```python
from build123d import *

# Parameters (mm, degrees)
HOLE_WIZARD_M32_D           = 2.5
HOLE_WIZARD_M32_DEPTH       = 8.5
HOLE_WIZARD_M32_CSINK_D     = 3.05
HOLE_WIZARD_M32_CSINK_ANGLE = 120
HOLE_WIZARD_M32_TIP         = 0.751075774
HOLE_WIZARD_1_D             = 3.3
HOLE_WIZARD_1_DEPTH         = 6
HOLE_WIZARD_1_CSINK_D       = 4.05
HOLE_WIZARD_1_CSINK_ANGLE   = 120
HOLE_WIZARD_1_TIP           = 0.991420021


with BuildPart() as part:
    # Эскиз2 → Повернуть1 (revolve)
    with BuildSketch(Plane(origin=(0, 0, 0), x_dir=(0, 0, -1), z_dir=(1, 0, 0))):
        Polygon((0, 0), (2, 0), (2, 0.01), (3, 0.01), (3, 8.01), (2, 8.01), (2, 25.01), (0, 25.01), align=None)
    revolve(axis=Axis((0, 0, 0), (0, 1, 0)))

    # Отверстие обработанное метчиком M32
    with Locations(Plane(origin=(0, 25.01, 0), x_dir=(-1, 0, 0), z_dir=(0, 1, 0))):
        with Locations((0, 0)):
            CounterSinkHole(HOLE_WIZARD_M32_D / 2, HOLE_WIZARD_M32_CSINK_D / 2, depth=HOLE_WIZARD_M32_DEPTH, counter_sink_angle=HOLE_WIZARD_M32_CSINK_ANGLE)
            with Locations((0, 0, -(HOLE_WIZARD_M32_DEPTH + HOLE_WIZARD_M32_TIP / 2))):  # 118° drill point
                Cone(0, HOLE_WIZARD_M32_D / 2, HOLE_WIZARD_M32_TIP, mode=Mode.SUBTRACT)

    # Отверстие обработанное метчиком 1
    with Locations(Plane.XZ):
        with Locations((0, 0)):
            CounterSinkHole(HOLE_WIZARD_1_D / 2, HOLE_WIZARD_1_CSINK_D / 2, depth=HOLE_WIZARD_1_DEPTH, counter_sink_angle=HOLE_WIZARD_1_CSINK_ANGLE)
            with Locations((0, 0, -(HOLE_WIZARD_1_DEPTH + HOLE_WIZARD_1_TIP / 2))):  # 118° drill point
                Cone(0, HOLE_WIZARD_1_D / 2, HOLE_WIZARD_1_TIP, mode=Mode.SUBTRACT)


solid = part.part
```
Input: part model. Units: mm. Frame: model coordinates. Give positions to 0.01 mm unless a question says otherwise; leave off trailing zeros. Order: outer loops, then holes, each group sorted by start corner. A loop starts at its lowest first (then second) coordinate and runs counter-clockwise, first axis right, second up. Notation, with made-up numbers: M 35.5,44.25 L 54.5,44.25 A17 cw 54.5,55.25 Z; hole C 1,74.25 d10. An arc over 180 degrees is marked long. One line per question, with ' | ' between items.
1) Ray query, L1, parallel to X at y = 4.8, z = 0; L2, parallel to X at y = 20.5, z = 0. Return the intervals inside material, ascending.
Filled in:
L1: x = -3 to -1.65, 1.65 to 3 | L2: x = -2 to -1.25, 1.25 to 2
2) Section D-D on y = 18.5. Output: boundary loops of the cut face in (x, z), and give its area (3 significant figures).
Filled in:
outline: C 0,0 d4; hole C 0,0 d2.5 | area: 7.66 mm2
3) Draft query along X for faces 1 (the face through (0, 4, 3)), 2 (the face through (-0.1, 6.8, -0.3)), 3 (the face through (2, 0.01, 1)), 4 (the face through (1.216, 3.149, 1.115)). Return one class per face: pulls with the +X half, pulls with the -X half, needs draft (parallel to the pull), parting line crosses it, or undercut.
Filled in:
face 1: parting line crosses it | face 2: undercut | face 3: needs draft | face 4: undercut
4) Section A-A on z = 2.4. Output: boundary loops of the cut face in (x, y).
Filled in:
outline: M -1.8,0.01 L 1.8,0.01 L 1.8,8.01 L -1.8,8.01 Z
5) Contact query for flat-ended pins moving along their axis: P1, Ø1, axis at y = 12, z = 0, coming from the -X side; P2, Ø2, axis at x = 0, z = 0, coming from the +Y side. Output: stop coordinate, or through.
Filled in:
P1: stops at x = -2 | P2: stops at y = 16.36
6) Section C-C on y = 2.25. Output: boundary loops of the cut face in (x, z).
Filled in:
outline: C 0,0 d6; hole C 0,0 d3.3
7) Section B-B on y = 11. Output: boundary loops of the cut face in (x, z), and give its area (3 significant figures).
Filled in:
outline: C 0,0 d4 | area: 12.6 mm2
